```python
from build123d import *

# Parameters (mm, degrees)
BOSS_EXTRUDE1_DEPTH = 2.4
SKETCH2_R           = 1.5
CUT_EXTRUDE1_DEPTH  = 2.4
THREAD2_PITCH       = 0.5


with BuildPart() as part:
    # Sketch1 → Boss-Extrude1 (new body)
    with BuildSketch(Plane(origin=(0, 0, 0), x_dir=(1, 0, 0), z_dir=(0, 1, 0))):
        Polygon((3.012171301, 1.710796321), (0.024492575, 3.464015028), (-2.987678726, 1.753218706), (-3.012171301, -1.710796321), (-0.024492575, -3.464015028), (2.987678726, -1.753218706), align=None)
    extrude(amount=BOSS_EXTRUDE1_DEPTH)

    # Sketch2 → Cut-Extrude1 (cut)
    with BuildSketch(Plane(origin=(0, 2.4, 0), x_dir=(1, 0, 0), z_dir=(0, 1, 0))):
        with Locations(Location((0, 0, 0), (0, 0, 270))):
            Circle(SKETCH2_R)
    extrude(amount=-CUT_EXTRUDE1_DEPTH, mode=Mode.SUBTRACT)

    # Thread2: the profile of Thread Profile2 profile screwed along a right-hand helix of 4.8 turns, 6 arcs to a turn; built about Z, then put on its axis
    thread2_z = Axis((0, 0, 0), (0, 0, 1))
    thread2_corners = [(1.4997, 0, -0.000173205), (1.770632938, 0, 0.156249999), (1.770632938, 0, 0.218749999), (1.4997, 0, 0.375173204)]
    with BuildLine(mode=Mode.PRIVATE) as thread2_profile:
        Line(thread2_corners[0], thread2_corners[1])
        Line(thread2_corners[1], thread2_corners[2])
        Line(thread2_corners[2], thread2_corners[3])
        Line(thread2_corners[3], thread2_corners[0])
    thread2_cap = Face(thread2_profile.wire())
    thread2_turn_angles = [0, 30, 60, 90, 120, 150, 180, 210, 240, 270, 300, 330, 360]
    thread2_turn_weights = [1, 0.8660254037844387, 1, 0.8660254037844387, 1, 0.8660254037844387, 1, 0.8660254037844387, 1, 0.8660254037844387, 1, 0.8660254037844387, 1]
    thread2_turn_rails = [Edge.make_bspline([Vector(p[0], p[1], 0).rotate(thread2_z, thread2_turn_angles[k]) / thread2_turn_weights[k] + Vector(0, 0, p[2] + THREAD2_PITCH * thread2_turn_angles[k] / 360) for k in range(13)], [0, 0, 0, 1, 1, 2, 2, 3, 3, 4, 4, 5, 5, 6, 6, 6], 2, thread2_turn_weights) for p in thread2_corners]
    thread2_turn_sides = [Face.make_surface_from_curves(thread2_turn_rails[p[0]], thread2_turn_rails[p[1]]) for p in [(0, 1), (1, 2), (2, 3), (3, 0)]]
    thread2_last_angles = [1440, 1470, 1500, 1530, 1560, 1590, 1620, 1650, 1680, 1704, 1728]
    thread2_last_weights = [1, 0.8660254037844387, 1, 0.8660254037844387, 1, 0.8660254037844387, 1, 0.8660254037844387, 1, 0.9135454576426009, 1]
    thread2_last_rails = [Edge.make_bspline([Vector(p[0], p[1], 0).rotate(thread2_z, thread2_last_angles[k]) / thread2_last_weights[k] + Vector(0, 0, p[2] + THREAD2_PITCH * thread2_last_angles[k] / 360) for k in range(11)], [0, 0, 0, 1, 1, 2, 2, 3, 3, 4, 4, 5, 5, 5], 2, thread2_last_weights) for p in thread2_corners]
    thread2_last_sides = [Face.make_surface_from_curves(thread2_last_rails[p[0]], thread2_last_rails[p[1]]) for p in [(0, 1), (1, 2), (2, 3), (3, 0)]]
    thread2 = Plane(origin=(0, 2.4, 0), x_dir=(-1, 0, 0), z_dir=(0, -1, 0)) * Solid(Shell([*[p.moved(Location((0, 0, THREAD2_PITCH * i))) for i in range(4) for p in thread2_turn_sides], *thread2_last_sides, thread2_cap, thread2_cap.rotate(thread2_z, 1728).moved(Location((0, 0, THREAD2_PITCH * 1728 / 360)))]))
    add(thread2, mode=Mode.SUBTRACT)


solid = part.part
```
CAD build for the part. Positions are in the model's coordinates, mm. Coordinates: 2 decimals unless noted, no trailing zeros. Order: outer loops, then holes, each group sorted by start corner. A loop starts at its lowest first (then second) coordinate and runs counter-clockwise, first axis right, second up. Notation, with made-up numbers: M 37,73.25 L 62,73.25 A15 cw 62,90.25 Z; hole C -34.5,-6 d8. An arc over 180 degrees is marked long. Answer as CSV lines item,"result".
1) Drill centre lines: L1, parallel to Z at x = 0, y = 0.75; L2, parallel to Z at x = 0.25, y = 0.5; L3, parallel to X at y = 0.3, z = -2. Where is each one in solid material? Low to high. Write a range as from..to.
Verdict:
L1,"-3.45..-1.54, 1.67..3.45"
L2,"-3.33..-1.68, 1.55..3.31"
L3,"-2.55..2.52"
2) Flat gauge pins, fed straight in: P1, Ø3.5, axis at x = 0, z = 0, coming from the -Y side; P2, Ø1, axis at y = 0.5, z = -1, coming from the -X side; P3, Ø1, axis at x = -1, y = 1, coming from the -Z side. Where does each tip first touch, or does it go through?
Verdict:
P1,"y = 0"
P2,"x = -3"
P3,"z = -3.17"
3) Cut at B-B (x = 2.75). List the corners of the cut face in (y, z).
Verdict:
outline,"M 0,-1.86 L 2.4,-1.86 L 2.4,1.89 L 0,1.89 Z"
4) Cut at A-A (z = 2). List the corners of the cut face in (x, y), then the cut area to 3 significant figures.
Verdict:
outline,"M -2.52,0 L 2.55,0 L 2.55,2.4 L -2.52,2.4 Z"
area,"12.2 mm2"
